Work out the finished part from the listing and answer in its coordinate system (mm). Face numbers are marked on the shaded views. Round coordinates to 2 decimals unless told otherwise and drop trailing zeros. Write each loop counter-clockwise with the first axis right and the second up, starting at its lowest first coordinate (ties: lowest second). Pieces come first, ordered by that corner, then holes. Notation, with made-up numbers: (20.25, -32.75) - (70.25, -32.75) arc R10 cw to (70.25, -16.75) - close; hole circle Ø6 at (87.25, 16.5). An arc over 180 degrees is marked (long way). Write item = value, one per line. Start each with the question number.
Autodesk Inventor part; units mm, degrees
ref_plane "YZ Plane" through (0, 0, 0) normal (1, 0, 0) x (0, 1, 0)
ref_plane "XZ Plane" through (0, 0, 0) normal (0, 1, 0) x (-1, 0, 0)
ref_plane "XY Plane" through (0, 0, 0) normal (0, 0, 1) x (1, 0, 0)
sketch "Sketch1" plane through (0, 0, 0) normal (0, 1, 0) x (-1, 0, 0)
  arc A0 (11.4609, -0.9477) -> (-11.4609, -0.9477) centre (0, 0) ccw
  arc A1 (-5.9796, -67.2325) -> (5.9796, -67.2325) centre (0, -66.738) ccw
  line L0 (11.4609, -0.9477) -> (5.9796, -67.2325)
  line L1 (-5.9796, -67.2325) -> (-11.4609, -0.9477)
  line L2 (7.2752, -67.3396) -> (12.7565, -1.0549)
  arc A2 (12.7565, -1.0549) -> (-12.7565, -1.0549) centre (0, 0) ccw
  line L3 (-12.7565, -1.0549) -> (-7.2752, -67.3396)
  arc A3 (-7.2752, -67.3396) -> (7.2752, -67.3396) centre (0, -66.738) ccw
  dimension "d0" = 23
  dimension "d1" = 12
  dimension "d2" = 66.511
  dimension "d6" = 1.3
extrude "Extrusion1" add sketch "Sketch1" along normal blind 6
properties part number "tandriem32Tnaar16T_lengte188"
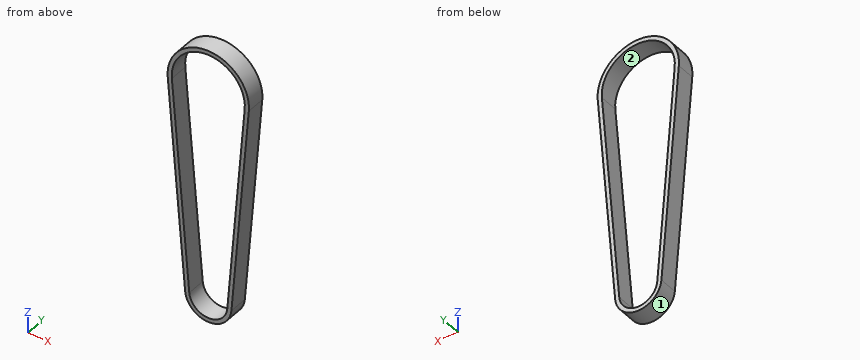
1. Consider line 1 (X direction, y = 2.25, z = 0); line 2 (X direction, y = 0.8, z = 8); line 3 (Z direction, x = -4.25, y = 1.3). Determine where each line is inside the solid, lowest interval first.
2. For a pull along Z with two mould halves and no side action, classify the marked faces 1 and 2 as released by +Z, released by -Z, zero draft, split by the parting line, or undercut.
3. Find section A-A on x = 0. Give the vertices of the cut face in (y, z).
4. Each of these flat-tipped pins is pushed along its axis until it touches: pin 1 (3 mm diameter, centred on x = -5, y = 4.5, fed in from -Z); pin 2 (1 mm diameter, centred on x = -7, y = 4.5, fed in from +Z). Where does it stop, or does it pass through?
5. Find section B-B on z = 0. Give the vertices of the cut face in (x, y), plus the area to 3 significant figures.
6. Find section C-C on y = 2.05. Give the vertices of the cut face in (x, z).
Answer key:
q1.line_1 = -12.8 to -11.5, 11.5 to 12.8
q1.line_2 = -9.99 to -8.26, 8.26 to 9.99
q1.line_3 = -72.67 to -70.97, 10.69 to 12.07
q2.face_1 = released by -Z
q2.face_2 = undercut
q3.outline = (0, -74.04) - (6, -74.04) - (6, -72.74) - (0, -72.74) - close; (0, 11.5) - (6, 11.5) - (6, 12.8) - (0, 12.8) - close
q4.pin_1 = -73.14
q4.pin_2 = 11.03
q5.outline = (-12.8, 0) - (-11.5, 0) - (-11.5, 6) - (-12.8, 6) - close; (11.5, 0) - (12.8, 0) - (12.8, 6) - (11.5, 6) - close
q5.area = 15.6 mm²
q6.outline = (-12.76, -1.05) - (-7.28, -67.34) arc R7.3 ccw to (7.28, -67.34) - (12.76, -1.05) arc R12.8 ccw (long way) to start; hole (-11.46, -0.95) - (-5.98, -67.23) arc R6 ccw to (5.98, -67.23) - (11.46, -0.95) arc R11.5 ccw (long way) to start
